from build123d import *

# Parameters (mm, degrees)
F0_R     = 5
F1_DEPTH = 6.035
F2_R     = 11.377245
F3_DEPTH = 12.07
F5_DEPTH = 12.07
F6_R     = 3.045388
F7_DEPTH = 25


with BuildPart() as f1:
    # F0 (on Right) → F1 (new body)
    with BuildSketch(Plane.YZ):
        Circle(F0_R)
    extrude(amount=-F1_DEPTH)

    # F2 (on face) → F3 (join)
    with BuildSketch(Plane.YZ):
        Circle(F2_R)
    extrude(amount=F3_DEPTH)

    # F4 (on face) → F5 (join)
    with BuildSketch(Plane.YZ.offset(12.07)):
        with BuildLine():
            ThreePointArc((11.377245, 0), (0, -11.377245), (-11.377245, 0))
            Line((-11.377245, 0), (-17.279675, -3.399281))
            Line((-17.279675, -3.399281), (-33.142988, -55.143889))
            Line((-33.142988, -55.143889), (0, -55.143889))
            Line((0, -55.143889), (33.142988, -55.143889))
            Line((33.142988, -55.143889), (17.279675, -3.399281))
            Line((17.279675, -3.399281), (11.377245, 0))
        make_face()
    extrude(amount=-F5_DEPTH)

    # F6 (on face) → F7 (cut)
    with BuildSketch(Plane(origin=(-6.035, 0, 0), x_dir=(0, -1, 0), z_dir=(-1, 0, 0))):
        Circle(F6_R)
    extrude(amount=-F7_DEPTH, mode=Mode.SUBTRACT)


solid = f1.part
Source: CAD feature listing. Evaluate the final solid. Frame: model axes, mm. A direction names the side the tool comes from. Round coordinates to 2 decimals unless told otherwise and drop trailing zeros. Write each loop counter-clockwise with the first axis right and the second up, starting at its lowest first coordinate (ties: lowest second). Pieces come first, ordered by that corner, then holes. Notation, with made-up numbers: (7.25, 1) - (47.25, 1) arc R21 ccw to (47.25, 6) - close; hole circle Ø2 at (64, -27). An arc over 180 degrees is marked (long way). Use CSV: the item, a comma, the result in double quotes. Start each with the question number.
(1) Cut plane D-D, the plane z = -39. Return loops of the section in (x, y), and give its area (3 significant figures).
(2) Material intervals for probe 1 along Z at (x, y) = (0.5, 0); probe 2 along X at (y, z) = (-16, -42); probe 3 along Z at (x, y) = (-1, -3.5), sorted ascending. Write a range as [from, to].
(3) First-contact query: pin 1 Ø1 at (y, z) = (5.5, -26) entering from -X; pin 2 Ø12 at (y, z) = (9.5, -3.5) entering from -X (3 decimals). Flat tips, straight axial feed; report the tip coordinate or a pass-through.
(4) Cut plane C-C, the plane x = -2.5. Return loops of the section in (y, z).
(5) Set-up query: faces 5 (the face through (-2.98, -1.08, -4.88)), 6 (the face through (5.951, 0.25, 11.374)). Return all of +Z, -Z, +X, -X, +Y, -Y with unobstructed straight access to the full face (end or side cutting, diameter ignored); none if empty.
(6) Cut plane A-A, the plane y = 0. Return loops of the section in (x, z) (3 decimals).
(7) Mould query, pull axis Z, two halves, no side actions, for faces 1 (the face through (6.12, -25.1, -28.91)), 2 (the face through (2.891, 2.245, 2.058)), 3 (the face through (6, 0, -55.144)), 4 (the face through (12.07, 0, -29)). Classes: pulls with the +Z half, pulls with the -Z half, needs draft (parallel to the pull), parting line crosses it, or undercut.
(8) Cut plane B-B, the plane x = 10.5. Return loops of the section in (y, z).
Geometry says:
1,outline,"(0, -28.19) - (12.07, -28.19) - (12.07, 28.19) - (0, 28.19) - close"
1,area,"681 mm²"
2,probe 1,"[-55.14, -3.05], [3.05, 11.38]"
2,probe 2,"[0, 12.07]"
2,probe 3,"[-3.57, 3.57]"
3,pin 1,"x = 0"
3,pin 2,"x = -6.035"
4,outline,"circle Ø10 at (0, 0); hole circle Ø6.09 at (0, 0)"
5,face 5,"-X"
5,face 6,"+Z, +X, -X"
6,outline,"(-6.035, -5) - (0, -5) - (0, -55.144) - (12.07, -55.144) - (12.07, -3.045) - (-6.035, -3.045) - close; (-6.035, 3.045) - (12.07, 3.045) - (12.07, 11.377) - (0, 11.377) - (0, 5) - (-6.035, 5) - close"
7,face 1,"pulls with the +Z half"
7,face 2,"undercut"
7,face 3,"pulls with the -Z half"
7,face 4,"needs draft"
8,outline,"(-33.14, -55.14) - (33.14, -55.14) - (17.28, -3.4) - (11.38, 0) arc R11.38 ccw to (-11.38, 0) - (-17.28, -3.4) - close; hole circle Ø6.09 at (0, 0)"
